Source: CAD feature listing. Evaluate the final solid. Frame: model axes, mm. Give positions to 0.01 mm unless a question says otherwise; leave off trailing zeros. Order: outer loops, then holes, each group sorted by start corner. A loop starts at its lowest first (then second) coordinate and runs counter-clockwise, first axis right, second up.
from build123d import *

# Parameters (mm, degrees)
SKETCH_1_W          = 640
SKETCH_1_H          = 595
EXTRUDE_1_DEPTH     = 15
SKETCH_2_R          = 2.5
CUT_EXTRUDE_1_DEPTH = 438.185601318
SKETCH_2_3_R        = 2.5
CUT_EXTRUDE_2_DEPTH = 438.185601318
SKETCH_3_R          = 40
CUT_EXTRUDE_3_DEPTH = 438.185601318


with BuildPart() as part:
    # ｽｹｯﾁ1 → ﾎﾞｽ - 押し出し1 (new body)
    with BuildSketch(Plane.XY):
        Rectangle(SKETCH_1_W, SKETCH_1_H)
    extrude(amount=EXTRUDE_1_DEPTH)

    # ｽｹｯﾁ2 → ｶｯﾄ - 押し出し1 (cut, through all)
    with BuildSketch(Plane.XY.offset(15)):
        with Locations((-270, 287.5)):
            Circle(SKETCH_2_R)
        with Locations((0, 287.5)):
            Circle(SKETCH_2_R)
        with Locations((270, 287.5)):
            Circle(SKETCH_2_R)
    cut_extrude_1 = extrude(amount=-CUT_EXTRUDE_1_DEPTH, mode=Mode.SUBTRACT)

    # ｽｹｯﾁ2<3> → ｶｯﾄ - 押し出し2 (cut, through all)
    with BuildSketch(Plane.XY.offset(15)):
        with Locations((-295, 247.5)):
            Circle(SKETCH_2_3_R)
        with Locations((-295, 0)):
            Circle(SKETCH_2_3_R)
        with Locations((-295, -247.5)):
            Circle(SKETCH_2_3_R)
    cut_extrude_2 = extrude(amount=-CUT_EXTRUDE_2_DEPTH, mode=Mode.SUBTRACT)

    # ﾐﾗｰ1: ｶｯﾄ - 押し出し1 across plane
    add(cut_extrude_1.mirror(Plane.ZX), mode=Mode.SUBTRACT)

    # ﾐﾗｰ2: ｶｯﾄ - 押し出し2 across plane
    add(cut_extrude_2.mirror(Plane(origin=(0, 0, 0), x_dir=(0, 0, 1), z_dir=(1, 0, 0))), mode=Mode.SUBTRACT)

    # ｽｹｯﾁ3 → ｶｯﾄ - 押し出し3 (cut, through all)
    with BuildSketch(Plane.XY.offset(15)):
        with Locations((200, -200)):
            Circle(SKETCH_3_R)
    extrude(amount=-CUT_EXTRUDE_3_DEPTH, mode=Mode.SUBTRACT)


solid = part.part
1) Section query A-A on y = -200. Output: boundary loops of the cut face in (x, z).
Checks:
outline: (-320, 0) - (160, 0) - (160, 15) - (-320, 15) - close; (240, 0) - (320, 0) - (320, 15) - (240, 15) - close
2) Pull-direction query (X, two-part tool) for faces 1 (the face through (168, -224, 8)), 2 (the face through (320, -4, 7)), 3 (the face through (-4, -297.5, 7)); classes: +X half, -X half, draft (parallel to the pull), parting line (faces both ways), or undercut.
Checks:
face 1: undercut
face 2: +X half
face 3: draft
3) First-contact query: pin 1 Ø4 at (x, y) = (295, 247.5) entering from -Z. Flat tip, straight axial feed; report the tip coordinate or a pass-through.
Checks:
pin 1: passes through
4) Ray query, L1, parallel to X at y = -247.5, z = 7; L2, parallel to Y at x = 270, z = 7; L3, parallel to Y at x = -295, z = 5.25. Return the intervals inside material, ascending.
Checks:
L1: x = -320 to -297.5, -292.5 to 292.5, 297.5 to 320
L2: y = -297.5 to -290, -285 to 285, 290 to 297.5
L3: y = -297.5 to -250, -245 to -2.5, 2.5 to 245, 250 to 297.5
5) Section query B-B on x = 200. Output: boundary loops of the cut face in (y, z), and give its area (4 significant figures).
Checks:
outline: (-297.5, 0) - (-240, 0) - (-240, 15) - (-297.5, 15) - close; (-160, 0) - (297.5, 0) - (297.5, 15) - (-160, 15) - close
area: 7,725 mm2
